Input: part model. Units: mm. Frame: model coordinates. Coordinates: 2 decimals unless noted, no trailing zeros. Loops run counter-clockwise (first coordinate to the right, second up) from the corner with the lowest first, then second, coordinate; pieces in that order, holes last. Notation, with made-up numbers: (-2.5, 75.5) -> (33.5, 75.5) arc R22 ccw to (33.5, 84.5) -> close; hole circle Ø9 at (-28, -23.75). An arc over 180 degrees is marked (long way). Answer as a JSON object with one key per item and string values.
from build123d import *

# Parameters (mm, degrees)
SKETCH1_R           = 107.95
SKETCH1_R_2         = 19.05
SKETCH1_W           = 2.921
SKETCH1_H           = 12.446
SKETCH1_W_2         = 12.446
SKETCH1_H_2         = 2.921
BOSS_EXTRUDE1_DEPTH = 3.175


with BuildPart() as part:
    # Sketch1 → Boss-Extrude1 (new body)
    with BuildSketch(Plane(origin=(0, 0, 0), x_dir=(1, 0, 0), z_dir=(0, 1, 0))):
        Circle(SKETCH1_R)
        with Locations((58.371664787, 58.371664787)):
            Circle(SKETCH1_R_2, mode=Mode.SUBTRACT)
        with Locations((58.371664787, -58.371664787)):
            Circle(SKETCH1_R_2, mode=Mode.SUBTRACT)
        with Locations((-58.371664787, -58.371664787)):
            Circle(SKETCH1_R_2, mode=Mode.SUBTRACT)
        with Locations((-58.371664787, 58.371664787)):
            Circle(SKETCH1_R_2, mode=Mode.SUBTRACT)
        with Locations((0, -94.742)):
            Rectangle(SKETCH1_W, SKETCH1_H, mode=Mode.SUBTRACT)
        with Locations((94.742, 0)):
            Rectangle(SKETCH1_W_2, SKETCH1_H_2, mode=Mode.SUBTRACT)
        with Locations((-94.742, 0)):
            Rectangle(SKETCH1_W_2, SKETCH1_H_2, mode=Mode.SUBTRACT)
        with Locations((0, 94.742)):
            Rectangle(SKETCH1_W, SKETCH1_H, mode=Mode.SUBTRACT)
    extrude(amount=-BOSS_EXTRUDE1_DEPTH)


solid = part.part
1. Pin query (flat end, axial travel): P1, Ø1, axis at x = 93.5, y = -1, coming from the +Z side; P2, Ø23, axis at x = 58.37, z = 58.37, coming from the +Y side; P3, Ø1, axis at y = -1, z = -96.5, coming from the -X side; P4, Ø1.6, axis at x = -96, y = -1, coming from the -Z side. Return the tip coordinate at first contact, or that it passes through.
Reply:
{"P1": "stops at z = 54.81", "P2": "passes through", "P3": "stops at x = -49.37", "P4": "stops at z = -50.89"}
2. Section query A-A (z = -70). Return loops of the section in (x, y) (3 decimals), plus the area to 3 significant figures.
Reply:
{"outline": "(-82.178, -3.175) -> (-73.461, -3.175) -> (-73.461, 0) -> (-82.178, 0) -> close; (-43.282, -3.175) -> (43.282, -3.175) -> (43.282, 0) -> (-43.282, 0) -> close; (73.461, -3.175) -> (82.178, -3.175) -> (82.178, 0) -> (73.461, 0) -> close", "area": "330 mm2"}
3. Section query B-B (y = -1.5). Count the separate pieces of the cut face and the enclosed holes in it, plus the area to 3 significant figures.
Reply:
{"separate pieces": "1", "enclosed holes": "8", "area": "31,900 mm2"}
4. Section query C-C (x = -35). Return loops of the section in (y, z) (3 decimals), plus the area to 3 significant figures.
Reply:
{"outline": "(-3.175, -102.119) -> (0, -102.119) -> (0, 102.119) -> (-3.175, 102.119) -> close", "area": "648 mm2"}
5. Line query: line 1 along X through (y, z) = (-2.4, 1) (3 decimals); line 2 along X through (y, z) = (-2.6, 74). Output: solid intervals per line, ascending.
Reply:
{"line 1": "x = -107.945 to -100.965, -88.519 to 88.519, 100.965 to 107.945", "line 2": "x = -78.6 to -69.26, -47.48 to 47.48, 69.26 to 78.6"}
6. Mould query, pull axis Z, two halves, no side actions, for faces 1 (the face through (39.34, -1.57, -59.21)), 2 (the face through (-79.56, -1.57, -72.96)), 3 (the face through (-2, -3.175, -2)). Classes: pulls with the +Z half, pulls with the -Z half, needs draft (parallel to the pull), parting line crosses it, or undercut.
Reply:
{"face 1": "undercut", "face 2": "parting line crosses it", "face 3": "needs draft"}
7. Section query D-D (z = 34). Return loops of the section in (x, y) (3 decimals), plus the area to 3 significant figures.
Reply:
{"outline": "(-102.456, -3.175) -> (102.456, -3.175) -> (102.456, 0) -> (-102.456, 0) -> close", "area": "651 mm2"}
